Source: CAD feature listing. Evaluate the final solid. Frame: model axes, mm. Face numbers are marked on the shaded views. A direction names the side the tool comes from. Round coordinates to 2 decimals unless told otherwise and drop trailing zeros. Write each loop counter-clockwise with the first axis right and the second up, starting at its lowest first coordinate (ties: lowest second). Pieces come first, ordered by that corner, then holes.
from build123d import *

# Parameters (mm, degrees)
F0_W     = 3
F0_H     = 80
F0_H_2   = 40
F0_H_3   = 79.9047601223
F1_DEPTH = 150
F3_DEPTH = 120
F4_SIZE  = 2
F5_SIZE  = 1
F6_SIZE  = 1
F7_SIZE  = 1


with BuildPart() as f1:
    # F0 (on Front) → F1 (new body)
    with BuildSketch(Plane.XZ):
        with Locations((-61.7444703951, 45)):
            Rectangle(F0_W, F0_H)
        Polygon((-60.2444703951, 5), (-63.2444703951, 5), (-63.2444703951, 0), (86.7555296049, 0), (86.7555296049, 5), (83.7555296049, 5), (23.7555296049, 5), (20.7555296049, 5), (-4.2444703951, 5), (-7.2444703951, 5), (-32.2444703951, 5), (-35.2444703951, 5), align=None)
        with Locations((-33.7444703951, 45)):
            Rectangle(F0_W, F0_H)
        with Locations((85.2555296049, 25)):
            Rectangle(F0_W, F0_H_2)
        with Locations((-5.7444703951, 45)):
            Rectangle(F0_W, F0_H)
        with Locations((22.2555296049, 44.9523800611)):
            Rectangle(F0_W, F0_H_3)
    extrude(amount=F1_DEPTH)

    # F2 (on face) → F3 (cut)
    with BuildSketch(Plane(origin=(-63.2444703951, 0, 0), x_dir=(0, -1, 0), z_dir=(-1, 0, 0))):
        Polygon((47.3553390593, 27.6776695297), (29.6776695297, 45.3553390593), (12, 27.6776695297), (29.6776695297, 10), align=None)
        Polygon((92.7106781187, 28.5361891277), (75.033008589, 46.2138586573), (57.3553390593, 28.5361891277), (75.033008589, 10.858519598), align=None)
        Polygon((138.066017178, 29.3947087257), (120.3883476483, 47.0723782553), (102.7106781187, 29.3947087257), (120.3883476483, 11.717039196), align=None)
        Polygon((69.60374879, 54.9267344821), (51.9260792603, 72.6044040117), (34.2484097307, 54.9267344821), (51.9260792603, 37.2490649524), align=None)
        Polygon((114.9590878493, 54.9267344821), (97.2814183197, 72.6044040117), (79.60374879, 54.9267344821), (97.2814183197, 37.2490649524), align=None)
    extrude(amount=-F3_DEPTH, mode=Mode.SUBTRACT)

    # F4
    f4_edges = [f1.edges().sort_by_distance(p)[0] for p in [
        (53.75553, -150, 5),
        (8.25553, -150, 5),
        (-19.74447, -150, 5),
        (-47.74447, -150, 5),
        (-47.74447, 0, 5),
        (-19.74447, 0, 5),
        (8.25553, 0, 5),
        (53.75553, 0, 5),
    ]]
    chamfer(f4_edges, length=F4_SIZE)

    # F5
    f5_edges = [f1.edges().sort_by_distance(p)[0] for p in [
        (-63.24447, -75, 0),
        (11.75553, -150, 0),
        (86.75553, -75, 0),
        (11.75553, 0, 0),
        (83.75553, -150, 25),
        (20.75553, -150, 44.95238),
        (-7.24447, -150, 45),
        (-35.24447, -150, 45),
        (-63.24447, -150, 42.5),
        (86.75553, -150, 22.5),
        (23.75553, -150, 44.95238),
        (-4.24447, -150, 45),
        (-32.24447, -150, 45),
        (-60.24447, -150, 45),
    ]]
    chamfer(f5_edges, length=F5_SIZE)

    # F6
    f6_edges = [f1.edges().sort_by_distance(p)[0] for p in [
        (83.75553, 0, 25),
        (86.75553, 0, 23),
        (23.75553, 0, 44.95238),
        (20.75553, 0, 44.95238),
        (-4.24447, 0, 45),
        (-7.24447, 0, 45),
        (-32.24447, 0, 45),
        (-35.24447, 0, 45),
        (-60.24447, 0, 45),
        (-63.24447, 0, 43),
    ]]
    chamfer(f6_edges, length=F6_SIZE)

    # F7
    f7_edges = [f1.edges().sort_by_distance(p)[0] for p in [
        (86.75553, -75, 45),
        (83.75553, -75, 45),
        (23.75553, -75, 84.90476),
        (20.75553, -75, 84.90476),
        (-4.24447, -75, 85),
        (-7.24447, -75, 85),
        (-32.24447, -75, 85),
        (-35.24447, -75, 85),
        (-60.24447, -75, 85),
        (-63.24447, -75, 85),
    ]]
    chamfer(f7_edges, length=F7_SIZE)


with BuildPart() as f1_1:
    # F8: moved
    add(f1.part.moved(Location((-12, 75, 0))))


solid = f1_1.part
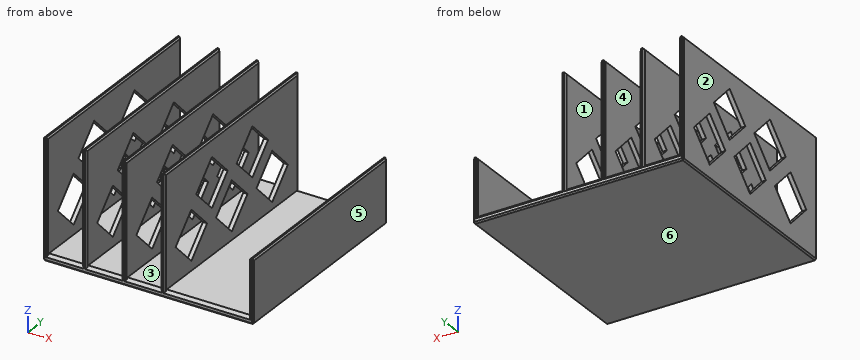
1) Pull-direction query (X, two-part tool) for the marked faces 3, 4, 5 and 6; classes: released by +X, released by -X, zero draft, split by the parting line, or undercut.
Taken from the geometry:
face 3: undercut
face 4: undercut
face 5: released by +X
face 6: zero draft
2) Contact query for flat-ended pins moving along their axis: P1, Ø0.5, axis at x = 10, y = -35.5, coming from the +Z side; P2, Ø6, axis at x = 49.5, y = 21.5, coming from the +Z side; P3, Ø1.1, axis at x = 73.5, y = 31, coming from the +Z side. Output: stop coordinate, or through.
Taken from the geometry:
P1: stops at z = 84.9
P2: stops at z = 5
P3: stops at z = 45
3) Section query B-B on x = -56. Return the cut outline in (y, z), then the cut area to 3 significant figures.
Taken from the geometry:
outline: (-75, 1) - (-74, 0) - (74, 0) - (75, 1) - (75, 3) - (73, 5) - (-73, 5) - (-75, 3) - close
area: 745 mm2
4) Section query A-A on z = 74.5. State how many separate pieces and enclosed holes the cut face has, then the cut area to 3 significant figures.
Taken from the geometry:
separate pieces: 4
enclosed holes: 0
area: 1,790 mm2
5) Material intervals for line 1 (X direction, y = -12, z = 18); line 2 (X direction, y = 11, z = 45.5); line 3 (Y direction, x = -45, z = 57.5), sorted ascending.
Taken from the geometry:
line 1: x = -75.24 to -72.24, -47.24 to -44.24, -19.24 to -16.24, 8.76 to 11.76, 71.76 to 74.76
line 2: x = -75.24 to -72.24, -47.24 to -44.24, -19.24 to -16.24, 8.76 to 11.76
line 3: y = -74.76 to -37.39, -7.18 to 7.97, 38.18 to 74.76
6) Reachability of the marked faces 1 and 2 from +Z, -Z, +X, -X, +Y, -Y: full face, straight path, thin tool, end or side. Return the list, or none.
Taken from the geometry:
face 1: +Z, +Y, -Y
face 2: +Z, -Z, -X, +Y, -Y
